Read the model definition and answer for the solid it produces. Units are mm, in the model's axes. A direction names the side the tool comes from. Round coordinates to 2 decimals unless told otherwise and drop trailing zeros. Loops run counter-clockwise (first coordinate to the right, second up) from the corner with the lowest first, then second, coordinate; pieces in that order, holes last. Notation, with made-up numbers: (0.25, 42) -> (22.25, 42) arc R21 ccw to (22.25, 76) -> close; hole circle Ø9 at (23.5, -23.5). An arc over 180 degrees is marked (long way). Put each result on its own line as item: value.
Autodesk Fusion 360 part; units mm, degrees
sketch "Sketch1" plane through (0, 0, 0) normal (0, 0, 1) x (1, 0, 0)
  line L0 (90, -18) -> (-90, -18)
  line L1 (-90, -18) -> (-90, 18)
  line L2 (-90, 18) -> (90, 18)
  line L3 (90, 18) -> (90, -18)
  line L4 (90, -18) -> (-90, 18) construction
  line L5 (-90, -18) -> (90, 18) construction
  line L6 (90, -13) -> (85.5, -13)
  line L7 (85.5, -13) -> (85.5, -3)
  line L8 (85.5, -3) -> (90, -3)
  line L9 (90, -3) -> (90, -13)
  line L10 (-90, -13) -> (-85.5, -13)
  line L11 (-85.5, -13) -> (-85.5, -3)
  line L12 (-85.5, -3) -> (-90, -3)
  line L13 (-90, -3) -> (-90, -13)
  line L14 (-98.0215, -0.75) -> (96.9785, -0.75) construction
  line L15 (55, -3) -> (30, -3)
  line L16 (30, -3) -> (30, 1.5)
  line L17 (30, 1.5) -> (55, 1.5)
  line L18 (55, 1.5) -> (55, -3)
  line L19 (55, -3) -> (30, 1.5) construction
  line L20 (30, -3) -> (55, 1.5) construction
  line L21 (-30, -3) -> (-55, -3)
  line L22 (-55, -3) -> (-55, 1.5)
  line L23 (-55, 1.5) -> (-30, 1.5)
  line L24 (-30, 1.5) -> (-30, -3)
  line L25 (-30, -3) -> (-55, 1.5) construction
  line L26 (-55, -3) -> (-30, 1.5) construction
  point P0 (42.5, -0.75)
  point P1 (-42.5, -0.75)
  dimension "d1" = 180
  dimension "d2" = 36
  dimension "d3" = 4.5
  dimension "d4" = 10
  dimension "d5" = 4.5
  dimension "d6" = 10
  dimension "d7" = 5
  dimension "d8" = 5
  dimension "d9" = 17.25
  dimension "d10" = 25
  dimension "d11" = 4.5
  dimension "d12" = 25
  dimension "d13" = 4.5
  dimension "d14" = 35
  dimension "d15" = 35
extrude "Extrude1" add sketch "Sketch1" along normal blind 4.5 contours L0 L1 L2 L3 L6 L7 L8 L10 L11 L12
Item 1: The part is cut by section B-B (y = -1.5). Determine the outline of the cut face in (x, z).
Derived:
outline: (-90, 0) -> (-55, 0) -> (-55, 4.5) -> (-90, 4.5) -> close; (-30, 0) -> (30, 0) -> (30, 4.5) -> (-30, 4.5) -> close; (55, 0) -> (90, 0) -> (90, 4.5) -> (55, 4.5) -> close
Item 2: Find the intervals of material crossed by line 1 along Y through (x, z) = (31, 0.25); line 2 along X through (y, z) = (-10, 0.95), in increasing order.
Derived:
line 1: y = -18 to -3, 1.5 to 18
line 2: x = -85.5 to 85.5
Item 3: Which of the six approach directions +Z, -Z, +X, -X, +Y, -Y give full straight-line access (tool end or side, diameter ignored) to faces 1 (the flat face through (-85.5, -8, 2)), 2 (the flat face through (-43, 1.5, 2)), 3 (the flat face through (88, -3, 2))?
Derived:
face 1: +Z, -Z, -X
face 2: +Z, -Z
face 3: +Z, -Z, +X
Item 4: The part is cut by section C-C (z = 1.75). Determine the outline of the cut face in (x, y).
Derived:
outline: (-90, -18) -> (90, -18) -> (90, -13) -> (85.5, -13) -> (85.5, -3) -> (90, -3) -> (90, 18) -> (-90, 18) -> (-90, -3) -> (-85.5, -3) -> (-85.5, -13) -> (-90, -13) -> close; hole (-55, -3) -> (-30, -3) -> (-30, 1.5) -> (-55, 1.5) -> close; hole (30, -3) -> (55, -3) -> (55, 1.5) -> (30, 1.5) -> close
Item 5: Flat-ended cylindrical pins translate along their axes: pin 1 Ø1.5 at (x, y) = (-64, -7.5) entering from -Z; pin 2 Ø1.3 at (y, z) = (-9.5, 1) entering from +X. Find the tip coordinate at first contact, or state that the pin passes through.
Derived:
pin 1: stops at z = 0
pin 2: stops at x = 85.5
Item 6: The part is cut by section A-A (x = -32.5). Determine the outline of the cut face in (y, z), then the cut area to 3 significant figures.
Derived:
outline: (-18, 0) -> (-3, 0) -> (-3, 4.5) -> (-18, 4.5) -> close; (1.5, 0) -> (18, 0) -> (18, 4.5) -> (1.5, 4.5) -> close
area: 142 mm^2
